Input: part model. Units: mm. Frame: model coordinates. A direction names the side the tool comes from. Give positions to 0.01 mm unless a question says otherwise; leave off trailing zeros. Loops run counter-clockwise (first coordinate to the right, second up) from the corner with the lowest first, then second, coordinate; pieces in that order, holes last. Notation, with made-up numbers: M 70,17 L 75,17 A18 cw 75,42 Z; hole C -11.5,-2 d7. An arc over 180 degrees is marked long. Return JSON: item names as keys, results as strings. Group by question number.
```python
from build123d import *

# Parameters (mm, degrees)
SKETCH_W     = 1000
SKETCH_H     = 500
PAD_DEPTH    = 100
SKETCH001_W  = 80
SKETCH001_H  = 80
PAD001_DEPTH = 420
SKETCH002_W  = 929.743311
SKETCH002_H  = 30.979035
PAD002_DEPTH = 500


with BuildPart() as part:
    # Sketch → Pad (new body)
    with BuildSketch(Plane.XZ):
        with Locations((500, 250)):
            Rectangle(SKETCH_W, SKETCH_H)
    extrude(amount=PAD_DEPTH)

    # Sketch001 → Pad001 (join)
    with BuildSketch(Plane.XZ):
        with Locations((42.294634, 460)):
            Rectangle(SKETCH001_W, SKETCH001_H)
        with Locations((40, 40)):
            Rectangle(SKETCH001_W, SKETCH001_H)
        with Locations((962.294634, 460)):
            Rectangle(SKETCH001_W, SKETCH001_H)
        with Locations((960, 40)):
            Rectangle(SKETCH001_W, SKETCH001_H)
    extrude(amount=PAD001_DEPTH)

    # Sketch002 (on Face16 of Pad001) → Pad002 (join)
    with BuildSketch(Plane(origin=(0, 0, 0), x_dir=(1, 0, 0), z_dir=(0, 0, -1))):
        with Locations((494.238269, 292.201278)):
            Rectangle(SKETCH002_W, SKETCH002_H)
    extrude(amount=-PAD002_DEPTH)


solid = part.part
```
Item 1: Section C-C, the plane y = -241.5. Return loops of the section in (x, z), then the cut area to 3 significant figures.
Item 2: Pull-direction query (Z, two-part tool) for faces 1 (the face through (959, -258, 80)), 2 (the face through (494, -67, 500)), 3 (the face through (80, -363, 39)); classes: pulls with the +Z half, pulls with the -Z half, needs draft (parallel to the pull), parting line crosses it, or undercut.
Item 3: Reachability of faces 4 (the face through (1000, -114, 67)), 5 (the face through (922.295, -187, 459)), 6 (the face through (80, -187, 39)) from +Z, -Z, +X, -X, +Y, -Y: full face, straight path, thin tool, end or side. Return the list, or none.
Item 4: Section D-D, the plane z = 67. Return loops of the section in (x, y), then the cut area to 3 significant figures.
Item 5: First-contact query: pin 1 Ø9.5 at (y, z) = (-291.5, 227) entering from -X; pin 2 Ø10 at (x, z) = (117.5, 121.5) entering from -Y; pin 3 Ø24 at (y, z) = (-338.5, 460.5) entering from -X. Flat tips, straight axial feed; report the tip coordinate or a pass-through.
Item 6: Section B-B, the plane x = 875. Return loops of the section in (y, z), then the cut area to 3 significant figures.
Item 7: Section A-A, the plane z = 387. Return loops of the section in (x, y).
Item 8: Material intervals for line 1 (Y direction, x = 845, z = 265); line 2 (X direction, y = -351, z = 466); line 3 (X direction, y = -95.5, z = 279), sorted ascending. Write a range as from..to.
Answer below:
{
 "1": {"outline": "M 0,0 L 80,0 L 80,80 L 0,80 Z; M 2.29,420 L 82.29,420 L 82.29,500 L 2.29,500 Z; M 920,0 L 1000,0 L 1000,80 L 920,80 Z; M 922.29,420 L 1002.29,420 L 1002.29,500 L 922.29,500 Z", "area": "25,600 mm^2"},
 "2": {"face 1": "undercut", "face 2": "pulls with the +Z half", "face 3": "needs draft"},
 "3": {"face 4": "-Z, +X, +Y, -Y", "face 5": "+Z", "face 6": "-Z"},
 "4": {"outline": "M 0,-420 L 80,-420 L 80,-307.69 L 920,-307.69 L 920,-420 L 1000,-420 L 1000,0 L 0,0 Z; hole M 80,-276.71 L 920,-276.71 L 920,-100 L 80,-100 Z", "area": "177,000 mm^2"},
 "5": {"pin 1": "x = 29.37", "pin 2": "y = -307.69", "pin 3": "x = 2.29"},
 "6": {"outline": "M -307.69,0 L -276.71,0 L -276.71,500 L -307.69,500 Z; M -100,0 L 0,0 L 0,500 L -100,500 Z", "area": "65,500 mm^2"},
 "7": {"outline": "M 0,-100 L 1000,-100 L 1000,0 L 0,0 Z; M 29.37,-307.69 L 959.11,-307.69 L 959.11,-276.71 L 29.37,-276.71 Z"},
 "8": {"line 1": "-307.69..-276.71, -100..0", "line 2": "2.29..82.29, 922.29..1002.29", "line 3": "0..1000"}
}
